Check sheet for the modelled part. Datum: model origin and axes. Units: mm. A direction names the side the tool comes from. Give positions to 0.01 mm unless a question says otherwise; leave off trailing zeros. Loops run counter-clockwise (first coordinate to the right, second up) from the corner with the lowest first, then second, coordinate; pieces in that order, holes last. Notation, with made-up numbers: M 69.25,4.25 L 112.25,4.25 A23 ccw 112.25,16.25 Z; hole C 70,69 d3. An arc over 180 degrees is marked long. Write each question's results on one line, items separated by ' | '. Start each with the question number.
1. Tool access check on faces 1 (the flat face through (2.5, 6, 26)), 2 (the flat face through (30, 21, 5)). Record the directions out of +Z, -Z, +X, -X, +Y, -Y that give a thin tool (end or side, any length) a straight path to the whole face; none if there is none.
2. Material ranges on line 1 along Y through (x, z) = (10, 19.5); line 2 along Z through (x, y) = (17.5, 5); line 3 along Z through (x, y) = (31, 19.5), recorded low to high.
3. Sectioned sample at C-C on x = 30. Record the cut outline in (y, z).
4. Sectioned sample at D-D on z = 23.5. Record the cut outline in (x, y), and give its area (3 significant figures).
5. Sectioned sample at B-B on y = 2. Record the cut outline in (x, z), and give its area (3 significant figures).
6. Go/stop test with flat-tipped pins: pin 1 (10 mm diameter, centred on x = 22, z = -10, fed in from +Y); pin 2 (11 mm diameter, centred on y = 19.5, z = 1, fed in from -X); pin 3 (2 mm diameter, centred on x = 31, y = 21, fed in from +Z). Record where each tip stops, or that it passes through.
7. Sectioned sample at A-A on x = 4. Record the cut outline in (y, z).
8. Draft check along Z on faces 3 (the flat face through (26, 12, 0)), 4 (the flat face through (30, 8, 2.4)), 5 (the flat face through (21, 0, 0)). Enter one of: pulls with the +Z half, pulls with the -Z half, needs draft (parallel to the pull), parting line crosses it, or undercut.
```python
from build123d import *

# Parameters (mm, degrees)
BOSS_EXTRUDE3_DEPTH      = 12
BOSS_EXTRUDE4_START      = -2
BOSS_EXTRUDE4_DEPTH      = 2
SKETCH3_W                = 6
SKETCH3_H                = 4.8
BOSS_EXTRUDE5_DEPTH      = 22
BOSS_EXTRUDE6_DEPTH      = 3
BOSS_EXTRUDE6_DEPTH_BACK = 1.5
SKETCH4_W                = 6
SKETCH4_H                = 10


with BuildPart() as part:
    # Sketch1 → Boss-Extrude3 (new body)
    with BuildSketch(Plane(origin=(0, 0, 0), x_dir=(1, 0, 0), z_dir=(0, 1, 0))):
        with BuildLine():
            Line((2.5, 27.386127875), (2.5, 25.377155081))
            ThreePointArc((2.5, 25.377155081), (25.5, 0), (2.5, -25.377155081))
            Line((2.5, -25.377155081), (2.5, -27.386127875))
            ThreePointArc((2.5, -27.386127875), (27.5, 0), (2.5, 27.386127875))
        make_face()
    extrude(amount=BOSS_EXTRUDE3_DEPTH)

    # Sketch2 → Boss-Extrude4 (add)
    with BuildSketch(Plane(origin=(0, 0, 0), x_dir=(1, 0, 0), z_dir=(0, 1, 0)).offset(BOSS_EXTRUDE4_START)):
        with BuildLine():
            Line((2.5, 27.386127875), (1.863636364, 20.415113507))
            ThreePointArc((1.863636364, 20.415113507), (20.5, 0), (1.863636364, -20.415113507))
            Line((1.863636364, -20.415113507), (2.5, -27.386127875))
            ThreePointArc((2.5, -27.386127875), (27.5, 0), (2.5, 27.386127875))
        make_face()
    extrude(amount=BOSS_EXTRUDE4_DEPTH)

    # Sketch3 → Boss-Extrude5 (add)
    with BuildSketch(Plane.XZ.offset(2)):
        with Locations((30, 0)):
            Rectangle(SKETCH3_W, SKETCH3_H)
    extrude(amount=-BOSS_EXTRUDE5_DEPTH)

    # Sketch4 → Boss-Extrude6 (add, two sides: drawn at the far end of the back side and taken through both)
    with BuildSketch(Plane(origin=(0, 20, 0), x_dir=(1, 0, 0), z_dir=(0, 1, 0)).offset(-BOSS_EXTRUDE6_DEPTH_BACK)):
        with Locations((30, 0)):
            Rectangle(SKETCH4_W, SKETCH4_H)
    extrude(amount=BOSS_EXTRUDE6_DEPTH + BOSS_EXTRUDE6_DEPTH_BACK)


solid = part.part
```
Output values:
1) face 1: +Z, -Z, -X, +Y | face 2: +Z, +X, -X, +Y, -Y
2) line 1: -2 to 0 | line 2: -21.21 to -18.55, 18.55 to 21.21 | line 3: -5 to 5
3) outline: M -2,-2.4 L 18.5,-2.4 L 18.5,-5 L 23,-5 L 23,5 L 18.5,5 L 18.5,2.4 L -2,2.4 Z
4) outline: M 2.15,-2 L 14.28,-2 L 14.28,12 L 9.9,12 L 9.9,0 L 2.15,0 Z | area: 76.9 mm2
5) outline: M 2.5,-27.39 A27.5 ccw 27.4,-2.4 L 33,-2.4 L 33,2.4 L 27.4,2.4 A27.5 ccw 2.5,27.39 L 2.5,25.38 A25.5 cw 2.5,-25.38 Z | area: 183 mm2
6) pin 1: y = 12 | pin 2: x = 27 | pin 3: z = 5
7) outline: M -2,-27.21 L 12,-27.21 L 12,-25.18 L 0,-25.18 L 0,-20.11 L -2,-20.11 Z; M -2,20.11 L 0,20.11 L 0,25.18 L 12,25.18 L 12,27.21 L -2,27.21 Z
8) face 3: needs draft | face 4: pulls with the +Z half | face 5: undercut
